The model under review builds one solid part; all positions refer to its coordinate system, in mm. Face numbers are marked on the shaded views. A direction names the side the tool comes from. Give positions to 0.01 mm unless a question says otherwise; leave off trailing zeros. Loops run counter-clockwise (first coordinate to the right, second up) from the corner with the lowest first, then second, coordinate; pieces in that order, holes last. Notation, with made-up numbers: M 60,18 L 78,18 A19 cw 78,38 Z; hole C 61.25,-6 d7. An arc over 180 degrees is marked long. Return JSON: item names as keys, results as strings.
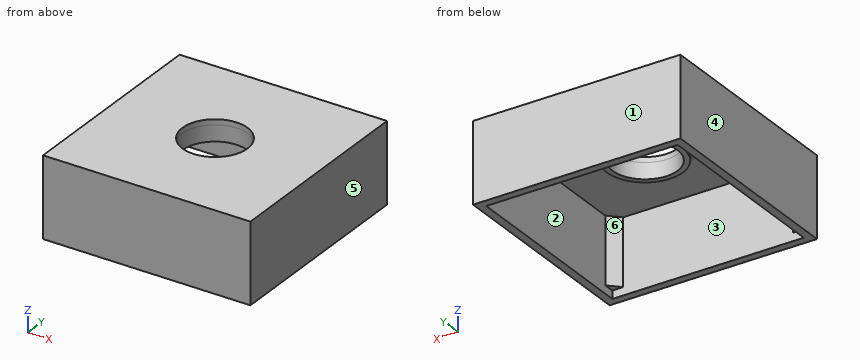
Autodesk Inventor part; units mm, degrees
ref_plane "YZ Plane" through (0, 0, 0) normal (1, 0, 0) x (0, 1, 0)
ref_plane "XZ Plane" through (0, 0, 0) normal (0, 1, 0) x (-1, 0, 0)
ref_plane "XY Plane" through (0, 0, 0) normal (0, 0, 1) x (1, 0, 0)
sketch "Sketch1" plane through (0, 0, 0) normal (0, 0, 1) x (1, 0, 0)
  line L0 (-11.7234, 6.1825) -> (24.1766, 6.1825)
  line L1 (24.1766, 6.1825) -> (24.1766, -29.7175)
  line L2 (24.1766, -29.7175) -> (-11.7234, -29.7175)
  line L3 (-11.7234, -29.7175) -> (-11.7234, 6.1825)
  line L4 (-13.2234, 7.6825) -> (25.6766, 7.6825)
  line L5 (25.6766, 7.6825) -> (25.6766, -31.2175)
  line L6 (25.6766, -31.2175) -> (-13.2234, -31.2175)
  line L7 (-13.2234, -31.2175) -> (-13.2234, 7.6825)
  point P0 (0, 0)
  dimension "d0" = 35.9
  dimension "d1" = 35.9
  dimension "d2" = 38.9
  dimension "d3" = 38.9
  dimension "d4" = 1.5
  dimension "d5" = 1.5
extrude "Extrusion1" add sketch "Sketch1" along normal blind 14
sketch "Sketch2" plane through (0, 0, 14) normal (0, 0, 1) x (1, 0, 0)
  line L0 (-13.2234, -31.2175) -> (-13.2234, 7.6825)
  line L1 (-13.2234, -31.2175) -> (25.6766, -31.2175)
  line L2 (-13.2234, 7.6825) -> (25.6766, 7.6825)
  line L3 (25.6766, 7.6825) -> (25.6766, -31.2175)
  line L4 (25.6766, -31.2175) -> (-13.2234, -31.2175)
  line L5 (-13.2234, -31.2175) -> (-13.2234, 7.6825)
  point P0 (0, 0)
extrude "Extrusion2" add sketch "Sketch2" along normal blind 1
sketch "Sketch3" plane through (0, 0, 15) normal (0, 0, 1) x (1, 0, 0)
  circle A0 centre (6.2266, -11.7675) radius 6.1
  line L0 (-13.2234, 7.6825) -> (-13.2234, -31.2175)
  line L1 (-13.2234, -31.2175) -> (25.6766, -31.2175)
  point P0 (0, 0)
  dimension "d10" = 12.2
  dimension "d11" = 19.45
  dimension "d12" = 19.45
  dimension "d13" = 38.9
extrude "Extrusion3" cut sketch "Sketch3" against normal blind 1
sketch "Sketch4" plane through (0, 0, 14) normal (0, 0, -1) x (-1, 0, 0)
  circle A0 centre (-6.2266, -11.7675) radius 6.1
  circle A1 centre (-6.2266, -11.7675) radius 7.1
  point P0 (0, 0)
  dimension "d16" = 14.2
extrude "Extrusion4" add sketch "Sketch4" along normal blind 3
fillet "Fillet1" radius 2 1 edges at (13.3266, -11.7675, 14)
sketch "Sketch5" plane through (0, 0, 14) normal (0, 0, -1) x (-1, 0, 0)
  line L0 (-24.1766, -29.7175) -> (11.7234, -29.7175)
  line L1 (11.7234, -29.7175) -> (9.7234, -29.7175)
  line L2 (9.7234, -29.7175) -> (11.7234, -27.7175)
  line L3 (11.7234, -29.7175) -> (11.7234, 6.1825)
  line L4 (11.7234, -27.7175) -> (11.7234, -29.7175)
  line L5 (11.7234, -29.7175) -> (11.7234, -27.7175)
  circle A0 centre (-6.2266, -11.7675) radius 6.1
  line L6 (11.7234, 6.1825) -> (11.7234, 4.1825)
  line L7 (9.7234, 6.1825) -> (11.7234, 6.1825)
  line L8 (11.7234, 4.1825) -> (9.7234, 6.1825)
  line L9 (-24.1766, 6.1825) -> (-22.1766, 6.1825)
  line L10 (-24.1766, 4.1825) -> (-24.1766, 6.1825)
  line L11 (-22.1766, 6.1825) -> (-24.1766, 4.1825)
  line L12 (-24.1766, -29.7175) -> (-24.1766, -27.7175)
  line L13 (-22.1766, -29.7175) -> (-24.1766, -29.7175)
  line L14 (-24.1766, -27.7175) -> (-22.1766, -29.7175)
  point P0 (0, 0)
  dimension "d20" = 2
  dimension "d21" = 45
  dimension "d24" = 360
extrude "Extrusion5" add sketch "Sketch5" along normal blind 12.5 contours L12 L14 L0 | L2 L3 L0 | L8 L7 L3 | L9 L11 L10
equation "\"d11\" = 0.5 * d13"
equation "\"d12\" = 0.5 * d13"
properties part number "lupa_camera_mount"
1) Tool access review of the marked faces 5 and 6: name each direction out of +Z, -Z, +X, -X, +Y, -Y from which nothing blocks a thin tool from reaching the whole face with its end or side.
From the geometry:
{"face 5": "+Z, -Z, +X, +Y, -Y", "face 6": "-Z"}
2) Insertion check: pin 1 (8 mm diameter, centred on x = 8, y = -1, fed in from -Z); pin 2 (1 mm diameter, centred on x = 23, y = -28.5, fed in from -Z); pin 3 (1.6 mm diameter, centred on x = -11, y = 5, fed in from -Z). Each pin has a flat end and moves straight along its axis. Give the tip position at first contact, or say it passes through.
From the geometry:
{"pin 1": "z = 11", "pin 2": "z = 1.5", "pin 3": "z = 0"}
3) The part is to be moulded in two halves that separate along X. For the marked faces 1, 2, 3 and 4, say which applies: released by +X, released by -X, zero draft, split by the parting line, or undercut.
From the geometry:
{"face 1": "zero draft", "face 2": "undercut", "face 3": "undercut", "face 4": "released by -X"}
4) Consider section D-D on y = 5.5. Write out the cut boundary in (x, z).
From the geometry:
{"outline": "M -13.22,0 L -11.72,0 L -11.72,1.5 L -10.41,1.5 L -10.41,14 L 22.86,14 L 22.86,1.5 L 24.18,1.5 L 24.18,0 L 25.68,0 L 25.68,15 L -13.22,15 Z"}
5) Consider section C-C on y = 1.5. Write out the cut boundary in (x, z), then the cut area to 3 significant figures.
From the geometry:
{"outline": "M -13.22,0 L -11.72,0 L -11.72,14 L 24.18,14 L 24.18,0 L 25.68,0 L 25.68,15 L -13.22,15 Z", "area": "80.9 mm²"}
6) Wall thickness on L1, parallel to Y at x = 21.5, z = 11.25; L2, parallel to X at y = -18, z = 10.5; L3, parallel to Y at x = 10, z = 12: over which ranges is each line inside the solid? List them lowest first. Write a range as from..to.
From the geometry:
{"L1": "-31.22..-29.72, 6.18..7.68", "L2": "-13.22..-11.72, 24.18..25.68", "L3": "-31.22..-29.72, -17.78..-16.56, -6.97..-5.75, 6.18..7.68"}
7) Consider section A-A on z = 9.75. Write out the cut boundary in (x, y), then the cut area to 3 significant figures.
From the geometry:
{"outline": "M -13.22,-31.22 L 25.68,-31.22 L 25.68,7.68 L -13.22,7.68 Z; hole M -11.72,-27.72 L -9.72,-29.72 L 22.18,-29.72 L 24.18,-27.72 L 24.18,4.18 L 22.18,6.18 L -9.72,6.18 L -11.72,4.18 Z", "area": "232 mm²"}
8) Consider section B-B on x = 20.5. Write out the cut boundary in (y, z), then the cut area to 3 significant figures.
From the geometry:
{"outline": "M -31.22,0 L -29.72,0 L -29.72,14 L 6.18,14 L 6.18,0 L 7.68,0 L 7.68,15 L -31.22,15 Z", "area": "80.9 mm²"}
